from build123d import *

# Parameters (mm, degrees)
BOSS_EXTRUDE1_DEPTH = 1219.2


with BuildPart() as part:
    # Sketch3 → Boss-Extrude1 (new body)
    with BuildSketch(Plane.XY):
        with BuildLine():
            Line((0, 15.24), (0, 92.202))
            ThreePointArc((0, 92.202), (-0.892738531, 94.357261469), (-3.048, 95.25))
            Line((-3.048, 95.25), (-6.35, 95.25))
            Line((-6.35, 95.25), (-6.35, -5.334))
            ThreePointArc((-6.35, -5.334), (-6.05242049, -6.05242049), (-5.334, -6.35))
            Line((-5.334, -6.35), (95.25, -6.35))
            Line((95.25, -6.35), (95.25, -3.048))
            ThreePointArc((95.25, -3.048), (94.357261469, -0.892738531), (92.202, 0))
            Line((92.202, 0), (15.24, 0))
            ThreePointArc((15.24, 0), (4.463692655, 4.463692655), (0, 15.24))
        make_face()
    extrude(amount=BOSS_EXTRUDE1_DEPTH)


solid = part.part
Here's how the part is built. I have some questions about the finished solid (model axes, mm). A direction names the side the tool comes from. Coordinates: 2 decimals unless noted, no trailing zeros. Write each loop counter-clockwise with the first axis right and the second up, starting at its lowest first coordinate (ties: lowest second). Pieces come first, ordered by that corner, then holes.
Item 1: If I drill on line 1 (X direction, y = 57, z = 669.5); line 2 (X direction, y = 11, z = 865), over which ranges is the centre line in solid material (lowest first)?
Item 2: I want a section at B-B on x = 54.5. Write out the boundary of the cut face in (y, z), and give its area (3 significant figures).
Item 3: I want a section at A-A on z = 884.5. Write out the boundary of the cut face in (x, y).
Item 4: On a 3-axis mill with a long thin cutter (end or side, diameter ignored), from which of +Z, -Z, +X, -X, +Y, -Y can I reach the whole of each face in a straight line? I mean faces 1 (the flat face through (54, 0, 601)), 2 (the flat face through (-1, 26, 1219.2)). Say none if no direction works.
Item 5: Will this pin go through, and if not, where does the flat tip stop? pin 1 (23 mm diameter, centred on y = 63, z = 889.5, fed in from +X).
Findings below:
1. line 1: x = -6.35 to 0
1. line 2: x = -6.35 to 0.6
2. outline: (-6.35, 0) - (0, 0) - (0, 1219.2) - (-6.35, 1219.2) - close
2. area: 7,740 mm2
3. outline: (-6.35, -5.33) arc R1.02 ccw to (-5.33, -6.35) - (95.25, -6.35) - (95.25, -3.05) arc R3.05 ccw to (92.2, 0) - (15.24, 0) arc R15.24 cw to (0, 15.24) - (0, 92.2) arc R3.05 ccw to (-3.05, 95.25) - (-6.35, 95.25) - close
4. face 1: +Z, -Z, +X, +Y
4. face 2: +Z, +X, -X, +Y, -Y
5. pin 1: stops at x = 0
